Geometry check sheet. Reference: the model listing, model coordinates, mm. Face numbers are marked on the shaded views. A direction names the side the tool comes from. Coordinates: 2 decimals unless noted, no trailing zeros. Loops run counter-clockwise (first coordinate to the right, second up) from the corner with the lowest first, then second, coordinate; pieces in that order, holes last.
from build123d import *

# Parameters (mm, degrees)
Y_KSEKLIK_EKSTR_ZYON1_DEPTH = 60
RADYUS1_RADIUS              = 30
RADYUS1_LENGTH              = 12
RADYUS2_RADIUS              = 30
RADYUS2_LENGTH              = 12
IZIM3_R                     = 12
KES_EKSTR_ZYON1_DEPTH       = 181.906004531
Y_KSEKLIK_EKSTR_ZYON2_DEPTH = 12
IZIM5_R                     = 20
IZIM5_R_2                   = 12
Y_KSEKLIK_EKSTR_ZYON3_DEPTH = 22
IZIM7_W                     = 12
IZIM7_H                     = 29.711788784
Y_KSEKLIK_EKSTR_ZYON6_DEPTH = 48
KES_EKSTR_ZYON2_DEPTH       = 162.92325206
IZIM9_R                     = 24
KES_EKSTR_ZYON3_DEPTH       = 211.376144164


with BuildPart() as part:
    # Çizim1 → Yükseklik-Ekstrüzyon1 (new body)
    with BuildSketch(Plane.XY):
        with BuildLine():
            Line((-102.970359754, 18.398808471), (-168.970359754, 18.398808471))
            Line((-168.970359754, 18.398808471), (-168.970359754, 30.398808471))
            Line((-168.970359754, 30.398808471), (-112.911485251, 30.398808471))
            ThreePointArc((-112.911485251, 30.398808471), (-78.970359754, 54.398808471), (-45.029234257, 30.398808471))
            Line((-45.029234257, 30.398808471), (11.029640246, 30.398808471))
            Line((11.029640246, 30.398808471), (11.029640246, 18.398808471))
            Line((11.029640246, 18.398808471), (-54.970359754, 18.398808471))
            ThreePointArc((-54.970359754, 18.398808471), (-78.970359754, 42.398808471), (-102.970359754, 18.398808471))
        make_face()
    extrude(amount=Y_KSEKLIK_EKSTR_ZYON1_DEPTH)

    # Radyus1: full round fillet: the end face becomes a half cylinder, R = half its width
    radyus1_face = Plane((-168.970359754, 24.398808471, 30), x_dir=(0, 1, 0), z_dir=(-1, 0, 0))  # on the end face: x along it, z out of the body
    radyus1_slab = radyus1_face.offset(-RADYUS1_RADIUS / 2) * Box(RADYUS1_LENGTH, 2 * RADYUS1_RADIUS, RADYUS1_RADIUS, mode=Mode.PRIVATE)  # the body's end, R deep
    radyus1_round = Plane((-138.970359754, 24.398808471, 30), x_dir=(-1, 0, 0), z_dir=(0, 1, 0)) * Cylinder(RADYUS1_RADIUS, RADYUS1_LENGTH, mode=Mode.PRIVATE)  # its axis R under the face
    add(radyus1_slab - radyus1_round, mode=Mode.SUBTRACT)

    # Radyus2: full round fillet: the end face becomes a half cylinder, R = half its width
    radyus2_face = Plane((11.029640246, 24.398808471, 30), x_dir=(0, 1, 0), z_dir=(1, 0, 0))  # on the end face: x along it, z out of the body
    radyus2_slab = radyus2_face.offset(-RADYUS2_RADIUS / 2) * Box(RADYUS2_LENGTH, 2 * RADYUS2_RADIUS, RADYUS2_RADIUS, mode=Mode.PRIVATE)  # the body's end, R deep
    radyus2_round = Plane((-18.970359754, 24.398808471, 30), x_dir=(1, 0, 0), z_dir=(0, 1, 0)) * Cylinder(RADYUS2_RADIUS, RADYUS2_LENGTH, mode=Mode.PRIVATE)  # its axis R under the face
    add(radyus2_slab - radyus2_round, mode=Mode.SUBTRACT)

    # Çizim3 → Kes-Ekstrüzyon1 (cut, through all)
    with BuildSketch(Plane(origin=(0, 30.398808471, 0), x_dir=(1, 0, 0), z_dir=(0, 1, 0))):
        with Locations(Location((-138.970359754, -30, 0), (0, 0, 270))):
            Circle(IZIM3_R)
        with Locations(Location((-18.970359754, -30, 0), (0, 0, 270))):
            Circle(IZIM3_R)
    extrude(amount=-KES_EKSTR_ZYON1_DEPTH, mode=Mode.SUBTRACT)

    # Çizim4 → Yükseklik-Ekstrüzyon2 (add)
    with BuildSketch(Plane(origin=(0, 0, 0), x_dir=(-1, 0, 0), z_dir=(0, 0, -1))):
        with BuildLine():
            Line((59.384707946, 99.821897357), (45.029234257, 30.398808471))
            Line((45.029234257, 30.398808471), (45.029234257, 18.398808471))
            Line((45.029234257, 18.398808471), (112.911485251, 18.398808471))
            Line((112.911485251, 18.398808471), (112.911485251, 30.398808471))
            Line((112.911485251, 30.398808471), (98.556011563, 99.821897357))
            ThreePointArc((98.556011563, 99.821897357), (78.970359754, 115.771929058), (59.384707946, 99.821897357))
        make_face()
    extrude(amount=-Y_KSEKLIK_EKSTR_ZYON2_DEPTH)

    # Çizim5 → Yükseklik-Ekstrüzyon3 (add)
    with BuildSketch(Plane.XY.offset(12)):
        with Locations(Location((-78.970359754, 95.771929058, 0), (0, 0, 168.316902305))):
            Circle(IZIM5_R)
        with Locations((-78.970359754, 95.771929058)):
            Circle(IZIM5_R_2, mode=Mode.SUBTRACT)
    extrude(amount=Y_KSEKLIK_EKSTR_ZYON3_DEPTH)

    # Çizim7 → Yükseklik-Ekstrüzyon6 (add)
    with BuildSketch(Plane.XY.offset(12)):
        with Locations((-78.970359754, 64.368074617)):
            Rectangle(IZIM7_W, IZIM7_H)
    extrude(amount=Y_KSEKLIK_EKSTR_ZYON6_DEPTH)

    # Çizim8 → Kes-Ekstrüzyon2 (cut, through all)
    with BuildSketch(Plane.ZY.offset(84.970359754)):
        Polygon((34, 76.693145029), (34, 79.223969009), (60, 79.223969009), (60, 53.895287169), align=None)
    extrude(amount=-KES_EKSTR_ZYON2_DEPTH, mode=Mode.SUBTRACT)

    # Çizim9 → Kes-Ekstrüzyon3 (cut, through all)
    with BuildSketch(Plane.XY.offset(12)):
        with Locations((-78.970359754, 18.398808471)):
            Circle(IZIM9_R)
    extrude(amount=-KES_EKSTR_ZYON3_DEPTH, mode=Mode.SUBTRACT)


solid = part.part
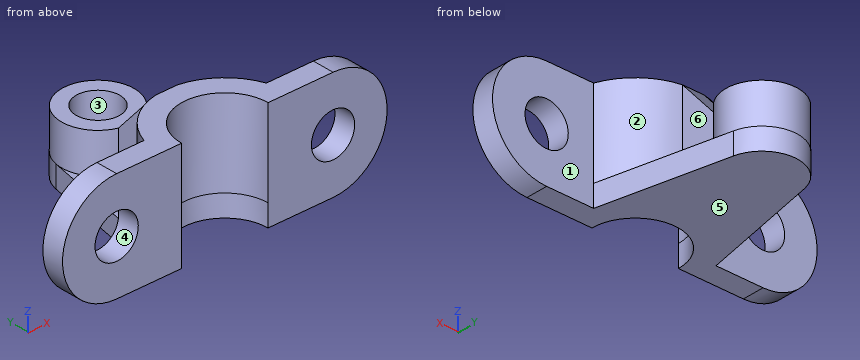
(1) Gauge pin test, flat ends, axial feed: pin 1 Ø18 at (y, z) = (67.5, 32.5) entering from +X; pin 2 Ø4 at (x, z) = (-118, 53.5) entering from +Y; pin 3 Ø3 at (y, z) = (49, 35.5) entering from -X. Record the tip position at first contact, or that the pin passes through.
Findings:
pin 1: stops at x = -72.97
pin 2: stops at y = 30.4
pin 3: stops at x = -100.16
(2) Scan lines: L1, parallel to Y at x = -85.5, z = 31; L2, parallel to X at y = 58, z = 46.5; L3, parallel to Y at x = -123.5, z = 24. Record each from-to range of solid material in increasing order.
Findings:
L1: y = 41.49 to 53.8, 76.87 to 85.7, 105.84 to 114.68
L2: x = -84.97 to -72.97
L3: y = 18.4 to 30.4
(3) Sectioned sample at C-C on z = 38.5. Record the cut outline in (x, y), and give its area (3 significant figures).
Findings:
outline: (-167.74, 18.4) - (-147.44, 18.4) - (-147.44, 30.4) - (-167.74, 30.4) - close; (-130.5, 18.4) - (-102.97, 18.4) arc R24 cw to (-54.97, 18.4) - (-27.44, 18.4) - (-27.44, 30.4) - (-45.03, 30.4) arc R36 ccw to (-72.97, 53.9) - (-72.97, 72.75) - (-84.97, 72.75) - (-84.97, 53.9) arc R36 ccw to (-112.91, 30.4) - (-130.5, 30.4) - close; (-10.5, 18.4) - (9.8, 18.4) - (9.8, 30.4) - (-10.5, 30.4) - close
area: 2,230 mm2
(4) Sectioned sample at D-D on x = -80. Record the cut outline in (y, z).
Findings:
outline: (42.38, 0) - (115.75, 0) - (115.75, 34) - (107.73, 34) - (107.73, 12) - (83.82, 12) - (83.82, 34) - (76.69, 34) - (53.9, 60) - (42.38, 60) - close
(5) Access from +Z, -Z, +X, -X, +Y, -Y to the whole of each face (thin tool, end or side, straight path). Record for the marked faces 1, 2 and 3.
Findings:
face 1: +Z, -Z, +X, +Y
face 2: +Z, +X
face 3: +Z
(6) Sectioned sample at A-A on y = 33. Record the cut outline in (x, z).
Findings:
outline: (-112.37, 0) - (-98.02, 0) - (-98.02, 60) - (-111.88, 60) - (-111.88, 12) - (-112.37, 12) - close; (-59.92, 0) - (-45.57, 0) - (-45.57, 12) - (-46.06, 12) - (-46.06, 60) - (-59.92, 60) - close
(7) Sectioned sample at B-B on z = 24.5. Record the cut outline in (x, y) (3 decimals).
Findings:
outline: (-168.462, 18.399) - (-149.636, 18.399) - (-149.636, 30.399) - (-168.462, 30.399) - close; (-128.305, 18.399) - (-102.97, 18.399) arc R24 cw to (-54.97, 18.399) - (-29.636, 18.399) - (-29.636, 30.399) - (-45.029, 30.399) arc R36 ccw to (-72.97, 53.895) - (-72.97, 76.693) arc R20 ccw (long way) to (-84.97, 76.693) - (-84.97, 53.895) arc R36 ccw to (-112.911, 30.399) - (-128.305, 30.399) - close; (-8.305, 18.399) - (10.521, 18.399) - (10.521, 30.399) - (-8.305, 30.399) - close; hole circle Ø24 at (-78.97, 95.772)
(8) Draft check along Z on the marked faces 4, 5 and 6. Enter one of: +Z half, -Z half, draft (parallel to the pull), parting line (faces both ways), or undercut.
Findings:
face 4: undercut
face 5: -Z half
face 6: draft
